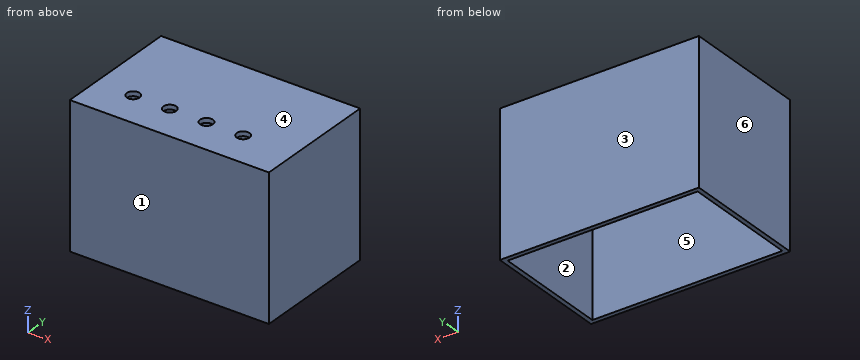
from build123d import *

# Parameters (mm, degrees)
SKETCH1_W           = 110
SKETCH1_H           = 70
BOSS_EXTRUDE1_DEPTH = 2.54
SKETCH4_W           = 110
SKETCH4_H           = 70
SKETCH4_W_2         = 105
SKETCH4_H_2         = 65
BOSS_EXTRUDE3_DEPTH = 76.2
SKETCH7_R           = 5.31
SKETCH7_R_2         = 2.77
BOSS_EXTRUDE5_DEPTH = 10
SKETCH9_R           = 3.55
CUT_EXTRUDE1_DEPTH  = 2.54


with BuildPart() as part:
    # Sketch1 → Boss-Extrude1 (new body)
    with BuildSketch(Plane.XY):
        with Locations((-3.180803055, -7.420155336)):
            Rectangle(SKETCH1_W, SKETCH1_H)
    extrude(amount=BOSS_EXTRUDE1_DEPTH)

    # Sketch4 → Boss-Extrude3 (add)
    with BuildSketch(Plane(origin=(0, 0, 0), x_dir=(-1, 0, 0), z_dir=(0, 0, -1))):
        with Locations((3.180803055, -7.420155336)):
            Rectangle(SKETCH4_W, SKETCH4_H)
        with Locations((3.180803055, -7.420155336)):
            Rectangle(SKETCH4_W_2, SKETCH4_H_2, mode=Mode.SUBTRACT)
    extrude(amount=BOSS_EXTRUDE3_DEPTH)

    # Sketch7 → Boss-Extrude5 (add)
    # profile 1 of 4: a face of its own
    with BuildSketch(Plane(origin=(0, 0, 0), x_dir=(-1, 0, 0), z_dir=(0, 0, -1))):
        with Locations(Location((-43.819196945, 17.579844664, 0), (0, 0, 180))):
            Circle(SKETCH7_R)
        with Locations((-43.819196945, 17.579844664)):
            Circle(SKETCH7_R_2, mode=Mode.SUBTRACT)
    # profile 2 of 4: a face of its own
    with BuildSketch(Plane(origin=(0, 0, 0), x_dir=(-1, 0, 0), z_dir=(0, 0, -1))):
        with Locations(Location((47.180803055, 17.579844664, 0), (0, 0, 180))):
            Circle(SKETCH7_R)
        with Locations((47.180803055, 17.579844664)):
            Circle(SKETCH7_R_2, mode=Mode.SUBTRACT)
    # profile 3 of 4: a face of its own
    with BuildSketch(Plane(origin=(0, 0, 0), x_dir=(-1, 0, 0), z_dir=(0, 0, -1))):
        with Locations(Location((47.180803055, -32.420155336, 0), (0, 0, 180))):
            Circle(SKETCH7_R)
        with Locations((47.180803055, -32.420155336)):
            Circle(SKETCH7_R_2, mode=Mode.SUBTRACT)
    # profile 4 of 4: a face of its own
    with BuildSketch(Plane(origin=(0, 0, 0), x_dir=(-1, 0, 0), z_dir=(0, 0, -1))):
        with Locations(Location((-43.819196945, -32.420155336, 0), (0, 0, 180))):
            Circle(SKETCH7_R)
        with Locations((-43.819196945, -32.420155336)):
            Circle(SKETCH7_R_2, mode=Mode.SUBTRACT)
    extrude(amount=BOSS_EXTRUDE5_DEPTH)

    # Sketch9 → Cut-Extrude1 (cut)
    with BuildSketch(Plane.XY.offset(2.54)):
        with Locations((23.169196945, -22.420155336)):
            Circle(SKETCH9_R)
        with Locations((2.919196945, -22.420155336)):
            Circle(SKETCH9_R)
        with Locations((-17.330803055, -22.420155336)):
            Circle(SKETCH9_R)
        with Locations((-37.580803055, -22.420155336)):
            Circle(SKETCH9_R)
    extrude(amount=-CUT_EXTRUDE1_DEPTH, mode=Mode.SUBTRACT)


solid = part.part
Model file for the job. Use its own axes, mm. Face numbers are marked on the shaded views. A direction names the side the tool comes from. Give positions to 0.01 mm unless a question says otherwise; leave off trailing zeros. Loops run counter-clockwise (first coordinate to the right, second up) from the corner with the lowest first, then second, coordinate; pieces in that order, holes last.
1) Saw through at C-C (z = -2). Count the separate pieces of the cut face and the enclosed holes in it, plus the area to 3 significant figures.
2) Flat gauge pins, fed straight in: pin 1 Ø4.5 at (x, y) = (-46, 17) entering from -Z; pin 2 Ø3 at (x, y) = (43.5, 18.5) entering from -Z; pin 3 Ø6.5 at (x, y) = (23.17, -22.42) entering from +Z. Where does each tip first touch, or does it go through?
3) Wall check: line 1 (X direction, y = -5, z = -5); line 2 (Y direction, x = -33, z = -41); line 3 (Z direction, x = -21, y = 22.5). Give the ranges that are in metal, low to high.
4) Saw through at D-D (x = -39). Write the cut outline in (y, z).
5) Saw through at A-A (z = -34). Write the cut outline in (x, y), plus the area to 3 significant figures.
6) Saw through at B-B (y = -14). Write the cut outline in (x, z).
7) Tool access for the marked faces 5 and 6: list every direction of +Z, -Z, +X, -X, +Y, -Y with a clear straight run to the whole face (end or side of a thin tool).
8) Pull direction Y, two halves, no side cores. Call the marked faces 1, 2, 3 and 4: +Y half, -Y half, draft (parallel to the pull), parting line (faces both ways), or undercut.
Answer block:
1. separate pieces: 5
1. enclosed holes: 5
1. area: 1,130 mm2
2. pin 1: stops at z = -10
2. pin 2: stops at z = 0
2. pin 3: passes through
3. line 1: x = -58.18 to -55.68, 49.32 to 51.82
3. line 2: y = -42.42 to -39.92, 25.08 to 27.58
3. line 3: z = 0 to 2.54
4. outline: (-42.42, -76.2) - (-39.92, -76.2) - (-39.92, 0) - (-25.67, 0) - (-25.67, 2.54) - (-42.42, 2.54) - close; (-19.17, 0) - (25.08, 0) - (25.08, -76.2) - (27.58, -76.2) - (27.58, 2.54) - (-19.17, 2.54) - close
5. outline: (-58.18, -42.42) - (51.82, -42.42) - (51.82, 27.58) - (-58.18, 27.58) - close; hole (-55.68, -39.92) - (49.32, -39.92) - (49.32, 25.08) - (-55.68, 25.08) - close
5. area: 875 mm2
6. outline: (-58.18, -76.2) - (-55.68, -76.2) - (-55.68, 0) - (49.32, 0) - (49.32, -76.2) - (51.82, -76.2) - (51.82, 2.54) - (-58.18, 2.54) - close
7. face 5: -Z
7. face 6: +Z, -Z, -X, +Y, -Y
8. face 1: -Y half
8. face 2: undercut
8. face 3: +Y half
8. face 4: draft
